Could you check a few things on this drawing? It's one solid part, dimensions in mm from its lowest x, y, z. A direction names the side the tool comes from. Give positions to 0.01 mm unless a question says otherwise; leave off trailing zeros. Order: outer loops, then holes, each group sorted by start corner. A loop starts at its lowest first (then second) coordinate and runs counter-clockwise, first axis right, second up. Notation, with made-up numbers: (-5, 14) - (40, 14) arc R23 cw to (40, 34) - close; hole circle Ø7 at (-22.5, -17). An arc over 180 degrees is marked (long way). Return JSON: item names as keys, results as strings.
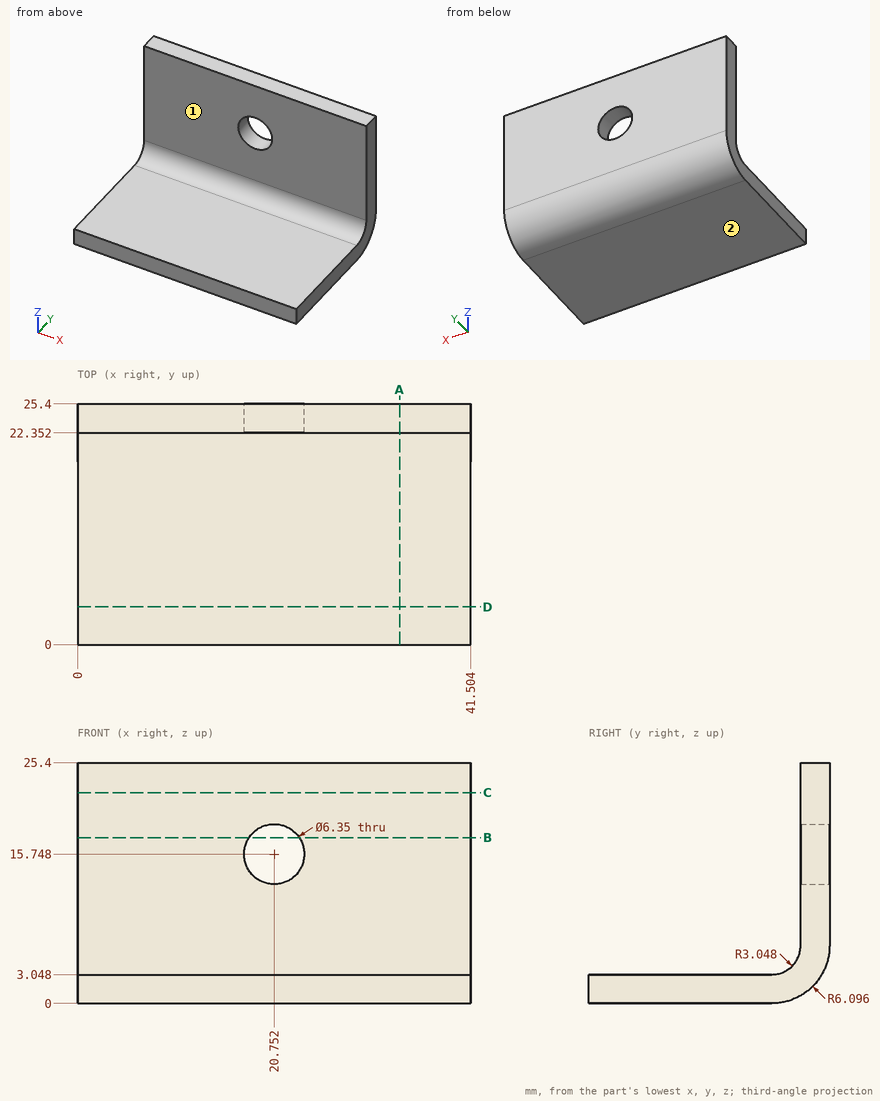
1. If I drill on L1, parallel to X at y = 23.5, z = 16; L2, parallel to Y at x = 37.5, z = 14.5; L3, parallel to Z at x = 13, y = 18.75, over which ranges is the centre line in solid material (lowest first)? Write a range as [from, to].
Checks:
{"L1": "[0, 17.59], [23.92, 41.5]", "L2": "[22.35, 25.4]", "L3": "[0, 3.05]"}
2. Suppose I cut it at D-D (y = 4). List the corners of the cut face in (x, z) for me.
Checks:
{"outline": "(0, 0) - (41.5, 0) - (41.5, 3.05) - (0, 3.05) - close"}
3. Suppose I cut it at A-A (x = 34). List the corners of the cut face in (y, z) for me.
Checks:
{"outline": "(0, 0) - (19.3, 0) arc R6.1 ccw to (25.4, 6.1) - (25.4, 25.4) - (22.35, 25.4) - (22.35, 6.1) arc R3.05 cw to (19.3, 3.05) - (0, 3.05) - close"}
4. Suppose I cut it at C-C (z = 22.25). List the corners of the cut face in (x, y) for me.
Checks:
{"outline": "(0, 22.35) - (41.5, 22.35) - (41.5, 25.4) - (0, 25.4) - close"}
5. For pin 1 Ø10 at (x, y) = (12, 4.5) entering from +Z; pin 2 Ø5 at (x, z) = (20.75, 15.75) entering from -Y; pin 3 Ø5 at (x, z) = (27.5, 3) entering from +Y, each with a flat end and sliding along its axis, tell me the tip position at first contact or that it passes through.
Checks:
{"pin 1": "z = 3.05", "pin 2": "through", "pin 3": "y = 25.37"}
6. On a 3-axis mill with a long thin cutter (end or side, diameter ignored), from which of +Z, -Z, +X, -X, +Y, -Y can I reach the whole of each face in a straight line? I mean the marked faces 1 and 2. Say none if no direction works.
Checks:
{"face 1": "+Z, +X, -X, -Y", "face 2": "-Z, +X, -X, +Y, -Y"}
7. Suppose I cut it at B-B (z = 17.5). List the corners of the cut face in (x, y) for me.
Checks:
{"outline": "(0, 22.35) - (18.1, 22.35) - (18.1, 25.4) - (0, 25.4) - close; (23.4, 22.35) - (41.5, 22.35) - (41.5, 25.4) - (23.4, 25.4) - close"}
